from build123d import *

# Parameters (mm, degrees)
F0_W     = 57.277
F0_H     = 16.002
F0_W_2   = 52.197
F0_H_2   = 10.922
F0_R     = 2.794
F1_DEPTH = 4.064
F2_DEPTH = 6.35
F3_R     = 3.81


with BuildPart() as f1:
    # F0 (on Top) → F1 (new body)
    with BuildSketch(Plane.XY):
        with BuildLine():
            Line((54.737, 17.272), (-2.54, 17.272))
            ThreePointArc((-2.54, 17.272), (-7.030128, 15.412128), (-8.89, 10.922))
            Line((-8.89, 10.922), (-8.89, 0))
            ThreePointArc((-8.89, 0), (-7.030128, -4.490128), (-2.54, -6.35))
            Line((-2.54, -6.35), (54.737, -6.35))
            ThreePointArc((54.737, -6.35), (59.227128, -4.490128), (61.087, 0))
            Line((61.087, 0), (61.087, 10.922))
            ThreePointArc((61.087, 10.922), (59.227128, 15.412128), (54.737, 17.272))
        make_face()
        with Locations((26.0985, 5.461)):
            Rectangle(F0_W, F0_H, mode=Mode.SUBTRACT)
        with Locations((26.0985, 5.461)):
            Rectangle(F0_W, F0_H)
        with Locations((26.0985, 5.461)):
            Rectangle(F0_W_2, F0_H_2, mode=Mode.SUBTRACT)
        with Locations((26.0985, 5.461)):
            Rectangle(F0_W_2, F0_H_2)
        with Locations((7.0485, 5.461)):
            Circle(F0_R, mode=Mode.SUBTRACT)
        with Locations((26.0985, 5.461)):
            Circle(F0_R, mode=Mode.SUBTRACT)
        with Locations((45.1485, 5.461)):
            Circle(F0_R, mode=Mode.SUBTRACT)
    extrude(amount=-F1_DEPTH)

    # F0 (on Top) → F2 (join)
    with BuildSketch(Plane.XY):
        with Locations((26.0985, 5.461)):
            Rectangle(F0_W, F0_H)
        with Locations((26.0985, 5.461)):
            Rectangle(F0_W_2, F0_H_2, mode=Mode.SUBTRACT)
    extrude(amount=F2_DEPTH)

    # F3
    f3_edges = [f1.edges().sort_by_distance(p)[0] for p in [
        (26.0985, -6.35, -4.064),
    ]]
    fillet(f3_edges, radius=F3_R)


solid = f1.part
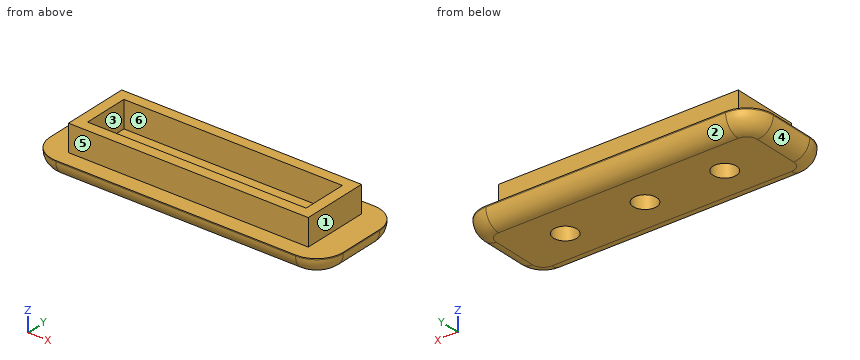
Geometry: final body of the model. Coordinates: model frame, mm. Face numbers are marked on the shaded views. A direction names the side the tool comes from. Round coordinates to 2 decimals unless told otherwise and drop trailing zeros. Loops run counter-clockwise (first coordinate to the right, second up) from the corner with the lowest first, then second, coordinate; pieces in that order, holes last. Notation, with made-up numbers: M 26,50.5 L 44,50.5 A17 ccw 44,73.5 Z; hole C 40,78.5 d7. An arc over 180 degrees is marked long. One line per question, with ' | ' between items.
(1) Cut plane C-C on y = 6.5. Return the cut outline in (x, z).
Check result:
outline: M -8.89,-0.25 A3.81 ccw -5.08,-4.06 L 4.45,-4.06 L 4.45,0 L 0,0 L 0,6.35 L -2.54,6.35 L -2.54,0 L -8.89,0 Z; M 9.64,-4.06 L 23.5,-4.06 L 23.5,0 L 9.64,0 Z; M 28.69,-4.06 L 42.55,-4.06 L 42.55,0 L 28.69,0 Z; M 47.74,-4.06 L 57.28,-4.06 A3.81 ccw 61.09,-0.25 L 61.09,0 L 54.74,0 L 54.74,6.35 L 52.2,6.35 L 52.2,0 L 47.74,0 Z
(2) Cut plane D-D on x = 16. Return the cut outline in (y, z).
Check result:
outline: M -6.35,-0.25 A3.81 ccw -2.54,-4.06 L 13.46,-4.06 A3.81 ccw 17.27,-0.25 L 17.27,0 L 13.46,0 L 13.46,6.35 L 10.92,6.35 L 10.92,0 L 0,0 L 0,6.35 L -2.54,6.35 L -2.54,0 L -6.35,0 Z
(3) Cut plane B-B on z = 3.75. Return the cut outline in (x, y), plus the area to 3 significant figures.
Check result:
outline: M -2.54,-2.54 L 54.74,-2.54 L 54.74,13.46 L -2.54,13.46 Z; hole M 0,0 L 52.2,0 L 52.2,10.92 L 0,10.92 Z | area: 346 mm2
(4) Pull-direction query (X, two-part tool) for the marked faces 3, 4, 5 and 6; classes: +X half, -X half, draft (parallel to the pull), parting line (faces both ways), or undercut.
Check result:
face 3: undercut | face 4: -X half | face 5: draft | face 6: undercut
(5) Material intervals for line 1 along X through (y, z) = (8, 4.25); line 2 along Y through (x, z) = (21.5, 5.5); line 3 along Z through (x, y) = (39, 7), sorted ascending. Write a range as from..to.
Check result:
line 1: x = -2.54..0, 52.2..54.74 | line 2: y = -2.54..0, 10.92..13.46 | line 3: z = -4.06..0
(6) Cut plane A-A on x = 46.5. Return the cut outline in (y, z), plus the area to 3 significant figures.
Check result:
outline: M -6.35,-0.25 A3.81 ccw -2.54,-4.06 L 3.02,-4.06 L 3.02,0 L 0,0 L 0,6.35 L -2.54,6.35 L -2.54,0 L -6.35,0 Z; M 7.91,-4.06 L 13.46,-4.06 A3.81 ccw 17.27,-0.25 L 17.27,0 L 13.46,0 L 13.46,6.35 L 10.92,6.35 L 10.92,0 L 7.91,0 Z | area: 102 mm2
(7) Contact query for flat-ended pins moving along their axis: P1, Ø1.9, axis at x = 16.5, z = 2, coming from the -Y side; P2, Ø5, axis at y = 7.5, z = 4, coming from the +X side; P3, Ø4.5, axis at x = 45.15, y = 5.46, coming from the -Z side; P4, Ø1.9, axis at y = 6, z = 3, coming from the -X side. Output: stop coordinate, or through.
Check result:
P1: stops at y = -2.54 | P2: stops at x = 54.74 | P3: passes through | P4: stops at x = -2.54
(8) Access query for the marked faces 1 and 2. Directions: +Z, -Z, +X, -X, +Y, -Y. A direction counts if a zero-diameter tool reaches every point of the face in a straight line with its end or side. Return the directions, or none.
Check result:
face 1: +Z, +X, +Y, -Y | face 2: -Z, +X, -X, +Y
